Work out the finished part from the listing and answer in its coordinate system (mm). Face numbers are marked on the shaded views. Round coordinates to 2 decimals unless told otherwise and drop trailing zeros. Loops run counter-clockwise (first coordinate to the right, second up) from the corner with the lowest first, then second, coordinate; pieces in that order, holes last. Notation, with made-up numbers: (-18.5, 20) - (32.5, 20) arc R15 ccw to (32.5, 36) - close; hole circle Ø10 at (55.25, 55). An arc over 180 degrees is marked (long way). Use CSV: the item, a comma, the result in double quotes. Start each with the question number.
from build123d import *

# Parameters (mm, degrees)
SKETCH1_R           = 12.7
BOSS_EXTRUDE1_DEPTH = 25.4
SKETCH2_R           = 4.075
CUT_EXTRUDE1_DEPTH  = 19.05
SKETCH3_R           = 1.25
CUT_EXTRUDE2_DEPTH  = 10


with BuildPart() as part:
    # Sketch1 → Boss-Extrude1 (new body)
    with BuildSketch(Plane(origin=(0, 0, 0), x_dir=(1, 0, 0), z_dir=(0, 1, 0))):
        Circle(SKETCH1_R)
    extrude(amount=BOSS_EXTRUDE1_DEPTH)

    # Sketch2 → Cut-Extrude1 (cut)
    with BuildSketch(Plane(origin=(0, 25.4, 0), x_dir=(1, 0, 0), z_dir=(0, 1, 0))):
        Circle(SKETCH2_R)
    extrude(amount=-CUT_EXTRUDE1_DEPTH, mode=Mode.SUBTRACT)

    # Sketch3 → Cut-Extrude2 (cut)
    with BuildSketch(Plane(origin=(0, 25.4, 0), x_dir=(1, 0, 0), z_dir=(0, 1, 0))):
        with Locations((0, 7.5)):
            Circle(SKETCH3_R)
        with Locations((6.495190528, -3.75)):
            Circle(SKETCH3_R)
        with Locations((-6.495190528, -3.75)):
            Circle(SKETCH3_R)
    extrude(amount=-CUT_EXTRUDE2_DEPTH, mode=Mode.SUBTRACT)


solid = part.part
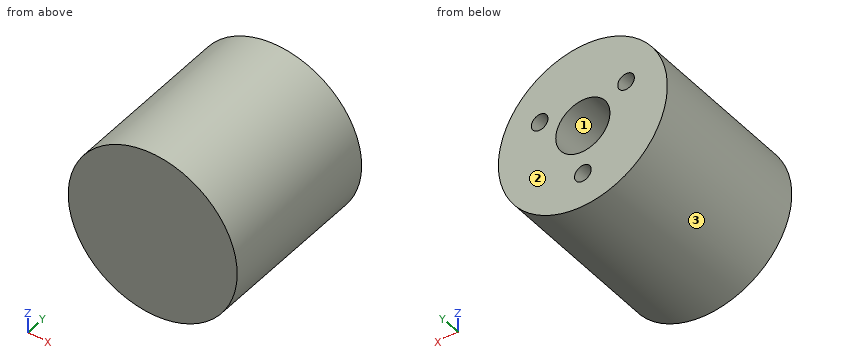
Item 1: A cutting plane is placed at A-A (z = 0). Determine the outline of the cut face in (x, y) (3 decimals), plus the area to 3 significant figures.
Item 2: The mould has two halves that part along Z. Classify the marked faces 1, 2 and 3: pulls with the +Z half, pulls with the -Z half, needs draft (parallel to the pull), parting line crosses it, or undercut.
Item 3: Find the intervals of material crossed by probe 1 along X at (y, z) = (15, 0) (3 decimals); probe 2 along X at (y, z) = (22.5, 3.75); probe 3 along Z at (x, y) = (3, 12.25), in increasing order. Write a range as [from, to].
Item 4: A cutting plane is placed at D-D (x = 6.25). Determine the outline of the cut face in (y, z), plus the area to 3 significant figures.
Item 5: Each of these flat-tipped pins is pushed along its axis until it touches: pin 1 Ø9.5 at (x, z) = (0, 0) entering from -Y; pin 2 Ø1.2 at (x, z) = (6, 3.5) entering from +Y; pin 3 Ø6 at (x, y) = (-5.5, 10.5) entering from -Z; pin 4 Ø3 at (x, y) = (7, 20.5) entering from -Z. Where does it stop, or does it pass through?
Item 6: A cutting plane is placed at B-B (x = 0). Determine the outline of the cut face in (y, z) (3 decimals), plus the area to 3 significant figures.
Item 7: A cutting plane is placed at C-C (y = 15). Determine the outline of the cut face in (x, z) (3 decimals).
Result sheet:
1,outline,"(-12.7, 0) - (12.7, 0) - (12.7, 25.4) - (4.075, 25.4) - (4.075, 6.35) - (-4.075, 6.35) - (-4.075, 25.4) - (-12.7, 25.4) - close"
1,area,"490 mm^2"
2,face 1,"undercut"
2,face 2,"needs draft"
2,face 3,"parting line crosses it"
3,probe 1,"[-12.7, -4.075], [4.075, 12.7]"
3,probe 2,"[-12.13, -7.75], [-5.25, -1.59], [1.59, 5.25], [7.75, 12.13]"
3,probe 3,"[-12.34, -2.76], [2.76, 12.34]"
4,outline,"(0, -11.06) - (25.4, -11.06) - (25.4, 2.52) - (15.4, 2.52) - (15.4, 4.98) - (25.4, 4.98) - (25.4, 11.06) - (0, 11.06) - close"
4,area,"537 mm^2"
5,pin 1,"y = 0"
5,pin 2,"y = 15.4"
5,pin 3,"z = -12.45"
5,pin 4,"z = -11.45"
6,outline,"(0, -12.7) - (25.4, -12.7) - (25.4, -8.75) - (15.4, -8.75) - (15.4, -6.25) - (25.4, -6.25) - (25.4, -4.075) - (6.35, -4.075) - (6.35, 4.075) - (25.4, 4.075) - (25.4, 12.7) - (0, 12.7) - close"
6,area,"465 mm^2"
7,outline,"circle Ø25.4 at (0, 0); hole circle Ø8.15 at (0, 0)"
